Geometry check sheet. Reference: drawing and pictorial views, mm from the part's lowest x, y, z. Give positions to 0.01 mm unless a question says otherwise; leave off trailing zeros. Loops run counter-clockwise (first coordinate to the right, second up) from the corner with the lowest first, then second, coordinate; pieces in that order, holes last. Notation, with made-up numbers: M 81,20 L 129,20 A28 ccw 129,56 Z; hole C 28,-7.75 d5. An arc over 180 degrees is marked long. Use CSV: the item, a comma, the result in double quotes.
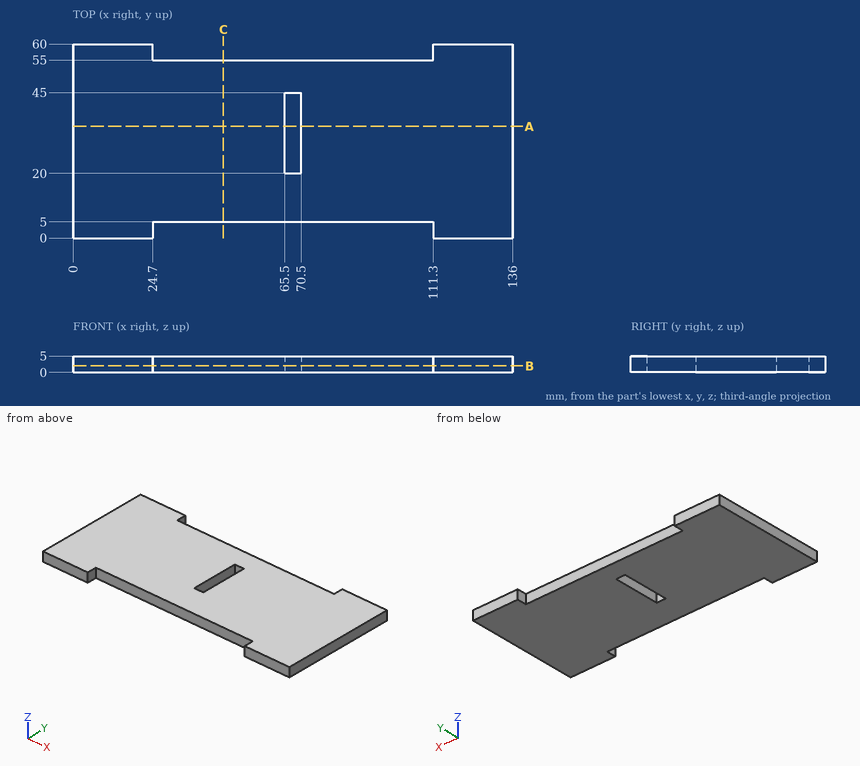
(1) Section check A-A on y = 34.5. Record the cut outline in (x, z), plus the area to 3 significant figures.
Calculated:
outline,"M 0,0 L 65.5,0 L 65.5,5 L 0,5 Z; M 70.5,0 L 136,0 L 136,5 L 70.5,5 Z"
area,"655 mm²"
(2) Section check B-B on z = 1.95. Record the cut outline in (x, y), plus the area to 3 significant figures.
Calculated:
outline,"M 0,0 L 24.7,0 L 24.7,5 L 111.3,5 L 111.3,0 L 136,0 L 136,60 L 111.3,60 L 111.3,55 L 24.7,55 L 24.7,60 L 0,60 Z; hole M 65.5,20 L 70.5,20 L 70.5,45 L 65.5,45 Z"
area,"7,170 mm²"
(3) Section check C-C on x = 46.5. Record the cut outline in (y, z), plus the area to 3 significant figures.
Calculated:
outline,"M 5,0 L 55,0 L 55,5 L 5,5 Z"
area,"250 mm²"
(4) Scan lines: L1, parallel to X at y = 26.5, z = 0.9; L2, parallel to X at y = 57, z = 1.25; L3, parallel to Y at x = 105.5, z = 0.45. Record each from-to range of solid material in increasing order. Write a range as from..to.
Calculated:
L1,"x = 0..65.5, 70.5..136"
L2,"x = 0..24.7, 111.3..136"
L3,"y = 5..55"
